The figure shows three views and two pictorial views of one solid part (mm, origin at its lowest corner). Answer the questions. A direction names the side the tool comes from. Round coordinates to 2 decimals unless told otherwise and drop trailing zeros. Loops run counter-clockwise (first coordinate to the right, second up) from the corner with the lowest first, then second, coordinate; pieces in that order, holes last. Notation, with made-up numbers: (51.5, 47.5) -> (88.5, 47.5) arc R23 cw to (88.5, 69.5) -> close; hole circle Ø7 at (44.5, 18.5). An arc over 180 degrees is marked (long way). Use a Markdown table: item, result. Add a question column.
Q1. Section C-C on y = 50 is taken. Give the vertices of the cut face in (x, z).
Q2. Consider line 1 (Y direction, x = 20.5, z = 0.75); line 2 (Y direction, x = 20.5, z = 4.85); line 3 (X direction, y = 43, z = 36.5). Determine where each line is inside the solid, lowest interval first.
Q3. Section D-D on y = 30 is taken. Give the vertices of the cut face in (x, z).
Q4. Section B-B on x = 4.5 is taken. Give the vertices of the cut face in (y, z), then the cut area to 3 significant figures.
Q5. Given pin 1 Ø15 at (y, z) = (43, 23) entering from -X; pin 2 Ø3.5 at (x, y) = (20.5, 10) entering from -Z; pin 3 Ø12 at (x, y) = (13.5, 19.5) entering from -Z; pin 4 Ø7 at (x, y) = (20.5, 50) entering from +Z, each flat-ended and moving along its own axis, determine where each tip first touches the part or whether it passes through.
Q6. Section A-A on z = 35.5 is taken. Give the vertices of the cut face in (x, y).
Q7. Which of the six approach directions +Z, -Z, +X, -X, +Y, -Y give full straight-line access (tool end or side, diameter ignored) to the marked faces 1, 2 and 3?
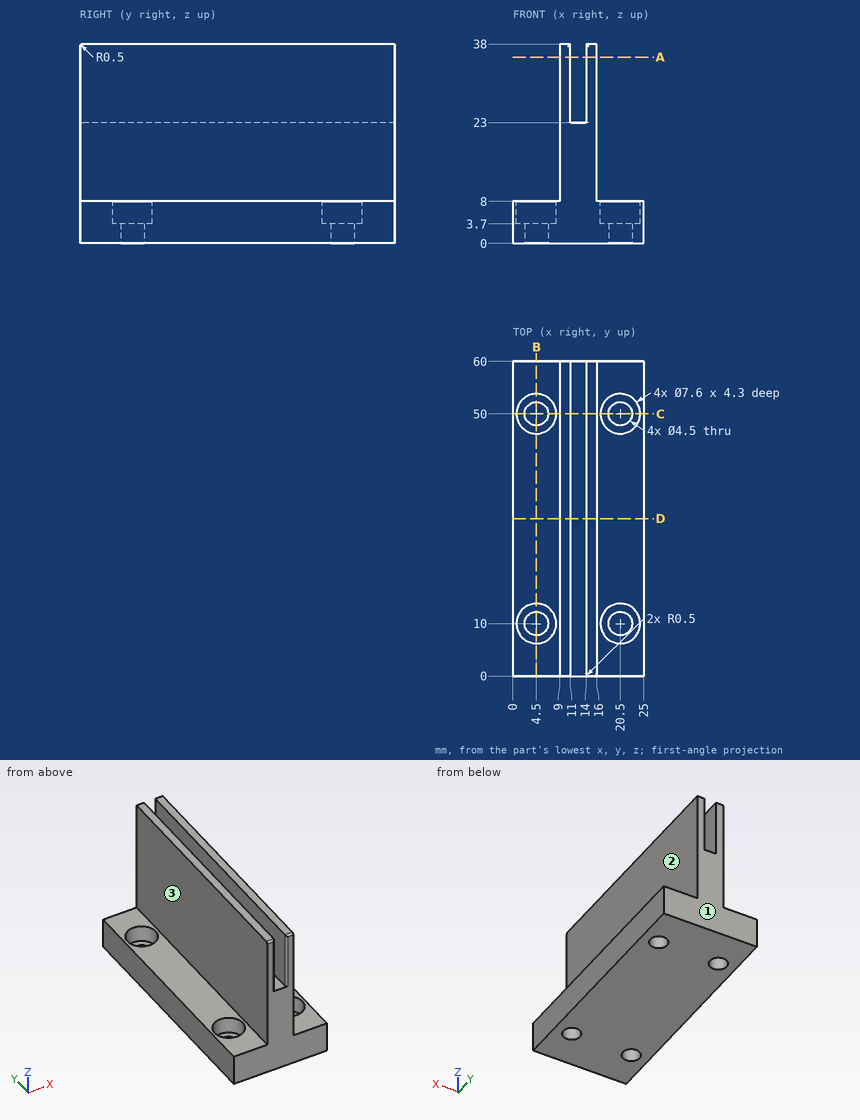
Checked values:
| question | item | result |
|---|---|---|
| 1 | outline | (0, 0) -> (2.25, 0) -> (2.25, 3.7) -> (0.7, 3.7) -> (0.7, 8) -> (0, 8) -> close; (6.75, 0) -> (18.25, 0) -> (18.25, 3.7) -> (16.7, 3.7) -> (16.7, 8) -> (16, 8) -> (16, 38) -> (14, 38) -> (14, 23) -> (11, 23) -> (11, 38) -> (9, 38) -> (9, 8) -> (8.3, 8) -> (8.3, 3.7) -> (6.75, 3.7) -> close; (22.75, 0) -> (25, 0) -> (25, 8) -> (24.3, 8) -> (24.3, 3.7) -> (22.75, 3.7) -> close |
| 2 | line 1 | y = 0 to 7.75, 12.25 to 47.75, 52.25 to 60 |
| 2 | line 2 | y = 0 to 6.2, 13.8 to 46.2, 53.8 to 60 |
| 2 | line 3 | x = 9 to 11, 14 to 16 |
| 3 | outline | (0, 0) -> (25, 0) -> (25, 8) -> (16, 8) -> (16, 38) -> (14, 38) -> (14, 23) -> (11, 23) -> (11, 38) -> (9, 38) -> (9, 8) -> (0, 8) -> close |
| 4 | outline | (0, 0) -> (7.75, 0) -> (7.75, 3.7) -> (6.2, 3.7) -> (6.2, 8) -> (0, 8) -> close; (12.25, 0) -> (47.75, 0) -> (47.75, 3.7) -> (46.2, 3.7) -> (46.2, 8) -> (13.8, 8) -> (13.8, 3.7) -> (12.25, 3.7) -> close; (52.25, 0) -> (60, 0) -> (60, 8) -> (53.8, 8) -> (53.8, 3.7) -> (52.25, 3.7) -> close |
| 4 | area | 381 mm2 |
| 5 | pin 1 | stops at x = 9 |
| 5 | pin 2 | passes through |
| 5 | pin 3 | stops at z = 0 |
| 5 | pin 4 | stops at z = 3.7 |
| 6 | outline | (9, 0) -> (10.5, 0) arc R0.5 ccw to (11, 0.5) -> (11, 60) -> (9, 60) -> close; (14, 0.5) arc R0.5 ccw to (14.5, 0) -> (16, 0) -> (16, 60) -> (14, 60) -> close |
| 7 | face 1 | +Z, -Z, +X, -X, +Y |
| 7 | face 2 | +Z, +X, +Y, -Y |
| 7 | face 3 | +Z, -X, +Y, -Y |
